Could you check a few things on this model? Use its own coordinates, in mm. Coordinates: 2 decimals unless noted, no trailing zeros. Write each loop counter-clockwise with the first axis right and the second up, starting at its lowest first coordinate (ties: lowest second). Pieces come first, ordered by that corner, then holes.
Item 1: If I drill on probe 1 along X at (y, z) = (-126, 7.75) (3 decimals); probe 2 along X at (y, z) = (-291, 17) (3 decimals); probe 3 along Y at (x, z) = (-500.5, 17.5), over which ranges is the centre line in solid material (lowest first)?
Item 2: I want a section at A-A on y = -44.45. Please give me the cut outline in (x, z) (3 decimals).
Item 3: I want a section at B-B on x = 465. Please give me the cut outline in (y, z), then the cut area to 3 significant figures.
Item 4: I want a section at D-D on z = 14.5. State how many separate pieces and enclosed holes the cut face has, then the cut area to 3 significant figures.
Item 5: For P1, Ø5.5, axis at x = 423, z = 8, coming from the +Y side; P2, Ø5, axis at y = -263.5, z = 9.5, coming from the +X side (3 decimals); P3, Ø1, axis at x = -138, y = -293.5, coming from the -Z side; P4, Ø5.5, axis at y = -298, z = 11.5, coming from the -X side (3 decimals), each with a flat end and sliding along its axis, tell me the tip position at first contact or that it passes through.
Item 6: I want a section at C-C on y = -282.5. Please give me the cut outline in (x, z) (3 decimals), then the cut area to 3 significant figures.
from build123d import *

# Parameters (mm, degrees)
F0_W     = 19.05
F0_H     = 152.4
F0_W_2   = 152.4
F0_H_2   = 19.05
F0_R     = 25.4
F1_DEPTH = 19.05


with BuildPart() as f1:
    # F0 (on Top) → F1 (new body)
    with BuildSketch(Plane.XY):
        Polygon((-511.175, 0), (-739.775, 0), (-739.775, -222.25), (-720.725, -222.25), (-720.725, -374.65), (-739.775, -374.65), (-739.775, -476.25), (739.775, -476.25), (739.775, -374.65), (720.725, -374.65), (720.725, -222.25), (739.775, -222.25), (739.775, -95.25), (739.775, 0), (511.175, 0), (511.175, -19.05), (358.775, -19.05), (358.775, 0), (-358.775, 0), (-358.775, -19.05), (-511.175, -19.05), align=None)
        with Locations((-243.416667, -298.45)):
            Rectangle(F0_W, F0_H, mode=Mode.SUBTRACT)
        with Locations((243.416667, -298.45)):
            Rectangle(F0_W, F0_H, mode=Mode.SUBTRACT)
        with Locations((-434.975, -123.825)):
            Rectangle(F0_W_2, F0_H_2, mode=Mode.SUBTRACT)
        with Locations((434.975, -123.825)):
            Rectangle(F0_W_2, F0_H_2, mode=Mode.SUBTRACT)
        with Locations((282.575, -44.45)):
            Circle(F0_R, mode=Mode.SUBTRACT)
    extrude(amount=F1_DEPTH)


solid = f1.part
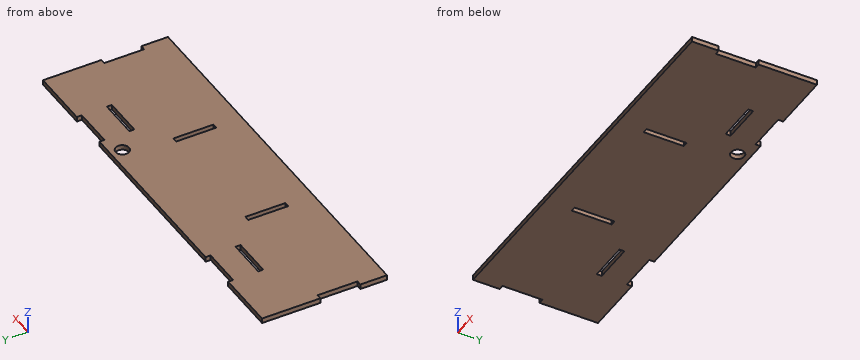
Response values:
1. probe 1: x = -739.775 to -511.175, -358.775 to 358.775, 511.175 to 739.775
1. probe 2: x = -720.725 to -252.942, -233.892 to 233.892, 252.942 to 720.725
1. probe 3: y = -476.25 to -133.35, -114.3 to -19.05
2. outline: (-739.775, 0) - (257.175, 0) - (257.175, 19.05) - (-739.775, 19.05) - close; (307.975, 0) - (739.775, 0) - (739.775, 19.05) - (307.975, 19.05) - close
3. outline: (-476.25, 0) - (-133.35, 0) - (-133.35, 19.05) - (-476.25, 19.05) - close; (-114.3, 0) - (-19.05, 0) - (-19.05, 19.05) - (-114.3, 19.05) - close
3. area: 8,350 mm2
4. separate pieces: 1
4. enclosed holes: 5
4. area: 679,000 mm2
5. P1: stops at y = -19.05
5. P2: stops at x = 720.725
5. P3: stops at z = 0
5. P4: stops at x = -720.725
6. outline: (-720.725, 0) - (-252.942, 0) - (-252.942, 19.05) - (-720.725, 19.05) - close; (-233.892, 0) - (233.892, 0) - (233.892, 19.05) - (-233.892, 19.05) - close; (252.942, 0) - (720.725, 0) - (720.725, 19.05) - (252.942, 19.05) - close
6. area: 26,700 mm2
